```python
from build123d import *

# Parameters (mm, degrees)
CUT_EXTRUDE2_DEPTH      = 2
CUT_EXTRUDE2_DEPTH_BACK = 1.81
SKETCH16_W              = 10.023590622
SKETCH16_H              = 2
SKETCH25_R              = 3
BOSS_EXTRUDE4_DEPTH     = 5
CHAMFER1_SIZE           = 0.3
SKETCH43_R              = 1.997454852
BOSS_EXTRUDE6_DEPTH     = 1


with BuildPart() as part:
    # Sketch2 → Revolve2 (revolve)
    with BuildSketch(Plane.XY):
        with BuildLine():
            ThreePointArc((-1.5, 6.225604788), (-3.652462654, 4.106847096), (-4.5, 1.207897271))
            Line((-4.5, 1.207897271), (-1.5, 1.213799777))
            Line((-1.5, 1.213799777), (-1.5, 6.225604788))
        make_face()
        Polygon((-1.5, 6.225604788), (-1.5, 1.213799777), (1.5, 1.219702283), (1.5, 6.225604788), align=None)
    revolve(axis=Axis((-4.5, 1.207897271, 0), (0.9999980644737863, 0.0019674980765590857, 0)))

    # Sketch16 → Cut-Extrude2 (cut, two sides: drawn at the far end of the back side and taken through both)
    with BuildSketch(Plane.ZY.offset(4.3).offset(-CUT_EXTRUDE2_DEPTH_BACK)):
        with Locations((0, 1.207897271)):
            Rectangle(SKETCH16_W, SKETCH16_H)
    extrude(amount=CUT_EXTRUDE2_DEPTH + CUT_EXTRUDE2_DEPTH_BACK, mode=Mode.SUBTRACT)

    # Sketch25 → Boss-Extrude4 (add)
    with BuildSketch(Plane(origin=(1.5, 0, 0), x_dir=(0, 0, -1), z_dir=(1, 0, 0))):
        with Locations(Location((0, 1.219702283, 0), (0, 0, 305.537696461))):
            Circle(SKETCH25_R)
    extrude(amount=BOSS_EXTRUDE4_DEPTH)

    # Chamfer1
    chamfer1_edges = [part.edges().sort_by_distance(p)[0] for p in [
        (6.5, 3.660902128, 1.743715377),
    ]]
    chamfer(chamfer1_edges, length=CHAMFER1_SIZE)

    # Sketch43 → Boss-Extrude6 (add)
    with BuildSketch(Plane(origin=(6.5, 0, 0), x_dir=(0, 0, -1), z_dir=(1, 0, 0))):
        with Locations((0, 1.219702283)):
            Circle(SKETCH43_R)
    extrude(amount=BOSS_EXTRUDE6_DEPTH)


solid = part.part
```
Geometry check sheet. Reference: the model listing, model coordinates, mm. A direction names the side the tool comes from. Give positions to 0.01 mm unless a question says otherwise; leave off trailing zeros. Write each loop counter-clockwise with the first axis right and the second up, starting at its lowest first coordinate (ties: lowest second). Pieces come first, ordered by that corner, then holes. Notation, with made-up numbers: (31, -3.75) -> (52, -3.75) arc R28 ccw to (52, 33.25) -> close; hole circle Ø5 at (89.5, -32.75). An arc over 180 degrees is marked (long way). Use one line per item in the form item = value.
Item 1: Sectioned sample at A-A on x = 4.5. Enter the section's corners in (y, z).
Results list:
outline = circle Ø6 at (1.22, 0)
Item 2: Access from +Z, -Z, +X, -X, +Y, -Y to the whole of each face (thin tool, end or side, straight path). Record for faces 4 (the cylindrical face through (6.99, -0.73, 0.43)), 5 (the flat face through (-3, 2.208, 0)).
Results list:
face_4 = +X
face_5 = +Z, -Z, -X
Item 3: Scan lines: line 1 (X direction, y = 0.5, z = -0.75); line 2 (X direction, y = 2, z = -2.5); line 3 (Y direction, x = 7.25, z = -0.75). Record each from-to range of solid material in increasing order.
Results list:
line_1 = -2.49 to 7.5
line_2 = -2.49 to 6.5
line_3 = -0.63 to 3.07
Item 4: Mould release check, pull along X, two halves, no side actions. Record for faces 1 (the flat face through (-3, 0.208, 0)), 2 (the flat face through (-2.49, 1, 0)), 3 (the flat face through (7.5, 1, 0)): released by +X, released by -X, zero draft, split by the parting line, or undercut.
Results list:
face_1 = zero draft
face_2 = released by -X
face_3 = released by +X
Item 5: Depth check by flat-ended pin: pin 1 Ø1.5 at (x, z) = (-3, -0.5) entering from -Y; pin 2 Ø1 at (x, y) = (6, -2) entering from +Z; pin 3 Ø4 at (x, z) = (-3, 2) entering from -Y. Enter the tip coordinate at first touch or a pass-through.
Results list:
pin_1 = -3.25
pin_2 = 1.27
pin_3 = -3.75
